from build123d import *

# Parameters (mm, degrees)
SKETCH_1_W          = 50
SKETCH_1_H          = 25
EXTRUDE_1_DEPTH     = 50
SKETCH_2_W          = 1.5
SKETCH_2_H          = 25
CUT_EXTRUDE_1_DEPTH = 44


with BuildPart() as part:
    # 草图1 → 拉伸1 (new body)
    with BuildSketch(Plane(origin=(0, 0, 0), x_dir=(1, 0, 0), z_dir=(0, 1, 0))):
        Rectangle(SKETCH_1_W, SKETCH_1_H)
    extrude(amount=EXTRUDE_1_DEPTH)

    # 草图2 → 切除-拉伸1 (cut)
    with BuildSketch(Plane(origin=(0, 50, 0), x_dir=(-1, 0, 0), z_dir=(0, 1, 0))):
        with Locations((-0.25, 0)):
            Rectangle(SKETCH_2_W, SKETCH_2_H)
        with Locations((2.25, 0)):
            Rectangle(SKETCH_2_W, SKETCH_2_H)
        with Locations((4.75, 0)):
            Rectangle(SKETCH_2_W, SKETCH_2_H)
        with Locations((7.25, 0)):
            Rectangle(SKETCH_2_W, SKETCH_2_H)
        with Locations((9.75, 0)):
            Rectangle(SKETCH_2_W, SKETCH_2_H)
        with Locations((12.25, 0)):
            Rectangle(SKETCH_2_W, SKETCH_2_H)
        with Locations((14.75, 0)):
            Rectangle(SKETCH_2_W, SKETCH_2_H)
        with Locations((17.25, 0)):
            Rectangle(SKETCH_2_W, SKETCH_2_H)
        with Locations((19.75, 0)):
            Rectangle(SKETCH_2_W, SKETCH_2_H)
        with Locations((22.25, 0)):
            Rectangle(SKETCH_2_W, SKETCH_2_H)
        with Locations((-2.75, 0)):
            Rectangle(SKETCH_2_W, SKETCH_2_H)
        with Locations((-5.25, 0)):
            Rectangle(SKETCH_2_W, SKETCH_2_H)
        with Locations((-7.75, 0)):
            Rectangle(SKETCH_2_W, SKETCH_2_H)
        with Locations((-10.25, 0)):
            Rectangle(SKETCH_2_W, SKETCH_2_H)
        with Locations((-12.75, 0)):
            Rectangle(SKETCH_2_W, SKETCH_2_H)
        with Locations((-15.25, 0)):
            Rectangle(SKETCH_2_W, SKETCH_2_H)
        with Locations((-17.75, 0)):
            Rectangle(SKETCH_2_W, SKETCH_2_H)
        with Locations((-20.25, 0)):
            Rectangle(SKETCH_2_W, SKETCH_2_H)
        with Locations((-22.75, 0)):
            Rectangle(SKETCH_2_W, SKETCH_2_H)
    extrude(amount=-CUT_EXTRUDE_1_DEPTH, mode=Mode.SUBTRACT)


solid = part.part
The listing builds one solid part. Answer for the finished solid, in the listing's coordinates (mm). Round coordinates to 2 decimals unless told otherwise and drop trailing zeros. Use a Markdown table: item, result. Add a question column.
1. Consider line 1 (Y direction, x = -22.5, z = -9.5). Determine where the line is inside the solid, lowest interval first.
2. Flat-ended cylindrical pins translate along their axes: P1, Ø0.8, axis at x = -7.5, z = -5.5, coming from the +Y side; P2, Ø1.2, axis at x = 20, z = -3, coming from the +Y side. Find the tip coordinate at first contact, or state that the pin passes through.
3. For a pull along X with two mould halves and no side action, classify faces 1 (the face through (-6, 25, 12.5)), 2 (the face through (3, 6, 0)) as +X half, -X half, draft (parallel to the pull), parting line (faces both ways), or undercut.
4. The part is cut by section A-A (y = 21). Give the number of separate pieces and of enclosed holes in the cut face, and give its area (4 significant figures).
Reported:
| question | item | result |
|---|---|---|
| 1 | line 1 | 0 to 6 |
| 2 | P1 | y = 6 |
| 2 | P2 | y = 50 |
| 3 | face 1 | draft |
| 3 | face 2 | undercut |
| 4 | separate pieces | 20 |
| 4 | enclosed holes | 0 |
| 4 | area | 537.5 mm^2 |
